Geometry: see drawing. Coordinates: mm, zero at the bounding-box minimum. A direction names the side the tool comes from. Round coordinates to 2 decimals unless told otherwise and drop trailing zeros. Order: outer loops, then holes, each group sorted by start corner. A loop starts at its lowest first (then second) coordinate and runs counter-clockwise, first axis right, second up. Notation, with made-up numbers: (77, 82.5) -> (100, 82.5) arc R24 cw to (100, 94.5) -> close; hole circle Ø9 at (-23, -0.75). An arc over 180 degrees is marked (long way). Use a Markdown table: item, result.
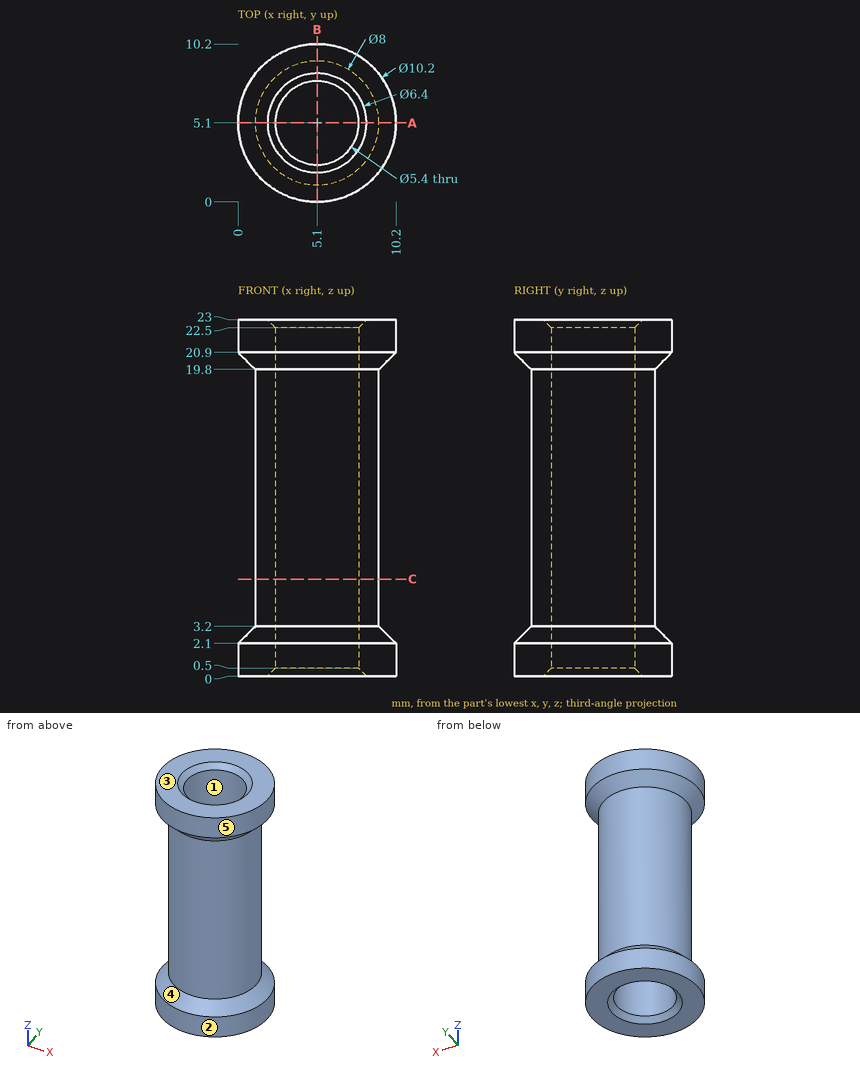
1) Draft query along Y for the marked faces 1, 2 and 3. Return one class per face: released by +Y, released by -Y, zero draft, split by the parting line, or undercut.
Answer key:
| item | result |
|---|---|
| face 1 | undercut |
| face 2 | split by the parting line |
| face 3 | zero draft |
2) Cut plane C-C on z = 6.25. Return loops of the section in (x, y), and give its area (3 significant figures).
Answer key:
| item | result |
|---|---|
| outline | circle Ø8 at (5.1, 5.1); hole circle Ø5.4 at (5.1, 5.1) |
| area | 27.4 mm^2 |
3) Contact query for flat-ended pins moving along their axis: P1, Ø5, axis at y = 3, z = 4.5, coming from the -X side; P2, Ø5, axis at y = 5, z = 16, coming from the -X side; P3, Ø6, axis at x = 4.5, z = 11.5, coming from the -Y side. Output: stop coordinate, or through.
Answer key:
| item | result |
|---|---|
| P1 | stops at x = 0.2 |
| P2 | stops at x = 1.1 |
| P3 | stops at y = 1.1 |
4) Cut plane A-A on y = 5.1. Return loops of the section in (x, z), and give its area (3 significant figures).
Answer key:
| item | result |
|---|---|
| outline | (0, 0) -> (1.9, 0) -> (2.4, 0.5) -> (2.4, 22.5) -> (1.9, 23) -> (0, 23) -> (0, 20.9) -> (1.1, 19.8) -> (1.1, 3.2) -> (0, 2.1) -> close; (7.8, 0.5) -> (8.3, 0) -> (10.2, 0) -> (10.2, 2.1) -> (9.1, 3.2) -> (9.1, 19.8) -> (10.2, 20.9) -> (10.2, 23) -> (8.3, 23) -> (7.8, 22.5) -> close |
| area | 71.0 mm^2 |
5) Set-up query: the marked faces 4 and 5. Return all of +Z, -Z, +X, -X, +Y, -Y with unobstructed straight access to the full face (end or side cutting, diameter ignored); none if empty.
Answer key:
| item | result |
|---|---|
| face 4 | none |
| face 5 | +Z, -Z |
6) Ray query, probe 1 along Y at (x, z) = (5.1, 15.5); probe 2 along Z at (x, y) = (7.25, 1.25); probe 3 along X at (y, z) = (3, 16.75). Return the intervals inside material, ascending.
Answer key:
| item | result |
|---|---|
| probe 1 | y = 1.1 to 2.4, 7.8 to 9.1 |
| probe 2 | z = 0 to 2.79, 20.21 to 23 |
| probe 3 | x = 1.7 to 3.4, 6.8 to 8.5 |
